```python
from build123d import *

# Parameters (mm, degrees)
F0_W     = 152.4
F0_H     = 50.8
F1_DEPTH = 31.7246
F2_DEPTH = 2.54
F3_DEPTH = 15.24


# Not quite as in the source:
# - a feature names something its author has since deleted; it is built from what else it names


with BuildPart() as f1:
    # F0 (on Top) → F1 (new body)
    with BuildSketch(Plane.XY):
        with Locations((76.2, 25.4)):
            Rectangle(F0_W, F0_H)
        with BuildLine():
            Line((139.6399507581, 16.4298143223), (139.6399507581, 6.0491856777))
            ThreePointArc((139.6399507581, 6.0491856777), (138.6121340696, 3.5678166885), (136.1307650805, 2.54))
            Line((136.1307650805, 2.54), (68.7885385865, 2.54))
            ThreePointArc((68.7885385865, 2.54), (66.7857906668, 3.167626223), (65.4994352256, 4.826))
            Line((65.4994352256, 4.826), (50.0925188645, 4.826))
            Line((50.0925188645, 4.826), (34.6856025033, 4.826))
            ThreePointArc((34.6856025033, 4.826), (28.3356025033, 11.176), (34.6856025033, 17.526))
            Line((34.6856025033, 17.526), (50.0925188645, 17.526))
            Line((50.0925188645, 17.526), (65.4549577669, 17.526))
            ThreePointArc((65.4549577669, 17.526), (66.7309106998, 19.2724454275), (68.7885385865, 19.939))
            Line((68.7885385865, 19.939), (136.1307650805, 19.939))
            ThreePointArc((136.1307650805, 19.939), (138.6121340696, 18.9111833115), (139.6399507581, 16.4298143223))
        make_face(mode=Mode.SUBTRACT)
    extrude(amount=F1_DEPTH)

    # F0 (on Top) → F2 (join)
    with BuildSketch(Plane.XY):
        with Locations((76.2, 25.4)):
            Rectangle(F0_W, F0_H)
        with BuildLine():
            Line((139.6399507581, 16.4298143223), (139.6399507581, 6.0491856777))
            ThreePointArc((139.6399507581, 6.0491856777), (138.6121340696, 3.5678166885), (136.1307650805, 2.54))
            Line((136.1307650805, 2.54), (68.7885385865, 2.54))
            ThreePointArc((68.7885385865, 2.54), (66.7857906668, 3.167626223), (65.4994352256, 4.826))
            Line((65.4994352256, 4.826), (50.0925188645, 4.826))
            Line((50.0925188645, 4.826), (34.6856025033, 4.826))
            ThreePointArc((34.6856025033, 4.826), (28.3356025033, 11.176), (34.6856025033, 17.526))
            Line((34.6856025033, 17.526), (50.0925188645, 17.526))
            Line((50.0925188645, 17.526), (65.4549577669, 17.526))
            ThreePointArc((65.4549577669, 17.526), (66.7309106998, 19.2724454275), (68.7885385865, 19.939))
            Line((68.7885385865, 19.939), (136.1307650805, 19.939))
            ThreePointArc((136.1307650805, 19.939), (138.6121340696, 18.9111833115), (139.6399507581, 16.4298143223))
        make_face(mode=Mode.SUBTRACT)
        with BuildLine():
            ThreePointArc((136.1307650805, 2.54), (138.6121340696, 3.5678166885), (139.6399507581, 6.0491856777))
            Line((139.6399507581, 6.0491856777), (139.6399507581, 16.4298143223))
            ThreePointArc((139.6399507581, 16.4298143223), (138.6121340696, 18.9111833115), (136.1307650805, 19.939))
            Line((136.1307650805, 19.939), (68.7885385865, 19.939))
            ThreePointArc((68.7885385865, 19.939), (66.7309106998, 19.2724454275), (65.4549577669, 17.526))
            Line((65.4549577669, 17.526), (50.0925188645, 17.526))
            ThreePointArc((50.0925188645, 17.526), (47.107835886, 11.176), (50.0925188645, 4.826))
            Line((50.0925188645, 4.826), (65.4994352256, 4.826))
            ThreePointArc((65.4994352256, 4.826), (66.7857906668, 3.167626223), (68.7885385865, 2.54))
            Line((68.7885385865, 2.54), (136.1307650805, 2.54))
        make_face()
        with BuildLine():
            ThreePointArc((92.2508400636, 8.0152933773), (89.0266334409, 11.2395), (92.2508400636, 14.4637066227))
            Line((92.2508400636, 14.4637066227), (110.0372854958, 14.4637066227))
            ThreePointArc((110.0372854958, 14.4637066227), (113.2614921185, 11.2395), (110.0372854958, 8.0152933773))
            Line((110.0372854958, 8.0152933773), (92.2508400636, 8.0152933773))
        make_face(mode=Mode.SUBTRACT)
        with BuildLine():
            Line((34.6856025033, 4.826), (50.0925188645, 4.826))
            ThreePointArc((50.0925188645, 4.826), (47.107835886, 11.176), (50.0925188645, 17.526))
            Line((50.0925188645, 17.526), (34.6856025033, 17.526))
            ThreePointArc((34.6856025033, 17.526), (28.3356025033, 11.176), (34.6856025033, 4.826))
        make_face()
    extrude(amount=-F2_DEPTH)

    # F0 (on Top) → F3 (join)
    with BuildSketch(Plane.XY):
        with BuildLine():
            Line((34.6856025033, 4.826), (50.0925188645, 4.826))
            ThreePointArc((50.0925188645, 4.826), (47.107835886, 11.176), (50.0925188645, 17.526))
            Line((50.0925188645, 17.526), (34.6856025033, 17.526))
            ThreePointArc((34.6856025033, 17.526), (28.3356025033, 11.176), (34.6856025033, 4.826))
        make_face()
    extrude(amount=F3_DEPTH)


solid = f1.part
```
Geometry check sheet. Reference: the model listing, model coordinates, mm. A direction names the side the tool comes from. Round coordinates to 2 decimals unless told otherwise and drop trailing zeros. Order: outer loops, then holes, each group sorted by start corner. A loop starts at its lowest first (then second) coordinate and runs counter-clockwise, first axis right, second up. Notation, with made-up numbers: (43, -10) - (69, -10) arc R24 ccw to (69, 20) - close; hole circle Ø8 at (27.25, -25.75). An arc over 180 degrees is marked (long way). Use a Markdown table: item, result. Add a question column.
1) Section check C-C (y = 13). Record the cut outline in (x, z).
2) Set-up check for faces 1 (the cylindrical face through (89.027, 11.169, -1.252)), 2 (the flat face through (75, 0, 15)), 3 (the cylindrical face through (66.81, 3.15, 15.64)): record each of +Z, -Z, +X, -X, +Y, -Y from which the full face is reachable in a straight line by a thin tool's end or side.
3) Mould release check, pull along Y, two halves, no side actions. Record for faces 4 (the flat face through (101, 8.015, -1)), 5 (the flat face through (152.4, 25, 15)), 6 (the flat face through (75, 50.8, 15)): released by +Y, released by -Y, zero draft, split by the parting line, or undercut.
4) Thickness scan on line 1 along Y through (x, z) = (96.5, 19); line 2 along Y through (x, z) = (62.5, 13); line 3 along Z through (x, y) = (111, 17). Record the ranges inside material, lowest first.
5) Section check D-D (z = 24). Record the cut outline in (x, y), then the cut area to 3 significant figures.
6) Section check B-B (x = 39). Record the cut outline in (y, z).
7) Section check A-A (z = 8). Record the cut outline in (x, y), then the cut area to 3 significant figures.
8) Gauge pin test, flat ends, axial feed: P1, Ø14, axis at x = 97.5, y = 13, coming from the +Z side; P2, Ø4, axis at x = 42, y = 11.5, coming from the +Z side. Record the tip position at first contact, or that the pin passes through.
Established:
| question | item | result |
|---|---|---|
| 1 | outline | (0, -2.54) - (89.55, -2.54) - (89.55, 0) - (47.31, 0) - (47.31, 15.24) - (28.6, 15.24) - (28.6, 31.72) - (0, 31.72) - close; (112.74, -2.54) - (152.4, -2.54) - (152.4, 31.72) - (139.64, 31.72) - (139.64, 0) - (112.74, 0) - close |
| 2 | face 1 | +Z, -Z |
| 2 | face 2 | +Z, -Z, +X, -X, -Y |
| 2 | face 3 | +Z |
| 3 | face 4 | undercut |
| 3 | face 5 | zero draft |
| 3 | face 6 | released by +Y |
| 4 | line 1 | 0 to 2.54, 19.94 to 50.8 |
| 4 | line 2 | 0 to 4.83, 17.53 to 50.8 |
| 4 | line 3 | -2.54 to 0 |
| 5 | outline | (0, 0) - (152.4, 0) - (152.4, 50.8) - (0, 50.8) - close; hole (34.69, 4.83) - (65.5, 4.83) arc R3.51 ccw to (68.79, 2.54) - (136.13, 2.54) arc R3.51 ccw to (139.64, 6.05) - (139.64, 16.43) arc R3.51 ccw to (136.13, 19.94) - (68.79, 19.94) arc R3.51 ccw to (65.45, 17.53) - (34.69, 17.53) arc R6.35 ccw to start |
| 5 | area | 6,010 mm2 |
| 6 | outline | (0, -2.54) - (50.8, -2.54) - (50.8, 31.72) - (17.53, 31.72) - (17.53, 15.24) - (4.83, 15.24) - (4.83, 31.72) - (0, 31.72) - close |
| 7 | outline | (0, 0) - (152.4, 0) - (152.4, 50.8) - (0, 50.8) - close; hole (50.09, 4.83) - (65.5, 4.83) arc R3.51 ccw to (68.79, 2.54) - (136.13, 2.54) arc R3.51 ccw to (139.64, 6.05) - (139.64, 16.43) arc R3.51 ccw to (136.13, 19.94) - (68.79, 19.94) arc R3.51 ccw to (65.45, 17.53) - (50.09, 17.53) arc R8.25 ccw to start |
| 7 | area | 6,240 mm2 |
| 8 | P1 | z = 31.72 |
| 8 | P2 | z = 15.24 |
